```python
from build123d import *

# Parameters (mm, degrees)
EXTRUDE_THIN1_DEPTH = 698.5
FILLET2_R           = 1.27


with BuildPart() as part:
    # Sketch1 → Extrude-Thin1 (new body)
    with BuildSketch(Plane.XY):
        with BuildLine():
            Line((0, 0), (-11.1125, 0))
            Line((-11.1125, 0), (-11.1125, 12.7))
            Line((-11.1125, 12.7), (-8.73125, 12.7))
            Line((-8.73125, 12.7), (-8.73125, 19.05))
            ThreePointArc((-8.73125, 19.05), (-21.768435997, 25.910734502), (-26.9875, 39.6875))
            ThreePointArc((-26.9875, 39.6875), (-24.662660076, 45.300160076), (-19.05, 47.625))
            Line((-19.05, 47.625), (-19.05, 50.8))
            Line((-19.05, 50.8), (-26.9875, 50.8))
            Line((-26.9875, 50.8), (-26.9875, 69.85))
            Line((-26.9875, 69.85), (1.5875, 69.85))
            Line((1.5875, 69.85), (1.5875, 68.58))
            Line((1.5875, 68.58), (-25.7175, 68.58))
            Line((-25.7175, 68.58), (-25.7175, 52.07))
            Line((-25.7175, 52.07), (-17.78, 52.07))
            Line((-17.78, 52.07), (-17.78, 46.232930181))
            ThreePointArc((-17.78, 46.232930181), (-23.291923576, 44.831587929), (-25.7175, 39.6875))
            ThreePointArc((-25.7175, 39.6875), (-20.440161015, 26.338097436), (-7.46125, 20.205828325))
            Line((-7.46125, 20.205828325), (-7.46125, 11.43))
            Line((-7.46125, 11.43), (-9.8425, 11.43))
            Line((-9.8425, 11.43), (-9.8425, 1.27))
            Line((-9.8425, 1.27), (0, 1.27))
            Line((0, 1.27), (0, 0))
        make_face()
    extrude(amount=-EXTRUDE_THIN1_DEPTH)

    # Fillet2
    fillet2_edges = [part.edges().sort_by_distance(p)[0] for p in [
        (-17.78, 52.07, -349.25),
        (-17.78, 46.232930181, -349.25),
        (-7.46125, 20.205828325, -349.25),
        (-7.46125, 11.43, -349.25),
        (-11.1125, 0, -349.25),
        (-11.1125, 12.7, -349.25),
        (-26.9875, 50.8, -349.25),
        (-26.9875, 69.85, -349.25),
    ]]
    fillet(fillet2_edges, radius=FILLET2_R)


solid = part.part
```
Read the model definition and answer for the solid it produces. Units are mm, in the model's axes. A direction names the side the tool comes from. Give positions to 0.01 mm unless a question says otherwise; leave off trailing zeros. Loops run counter-clockwise (first coordinate to the right, second up) from the corner with the lowest first, then second, coordinate; pieces in that order, holes last.
Item 1: Find the intervals of material crossed by line 1 along Y through (x, z) = (-7, -520); line 2 along Y through (x, z) = (-21.25, -264); line 3 along Y through (x, z) = (-19, -640), in increasing order.
Item 2: Each of these flat-tipped pins is pushed along its axis until it touches: pin 1 Ø4 at (y, z) = (50.5, -372) entering from +X; pin 2 Ø1.6 at (y, z) = (49, -371.5) entering from -X; pin 3 Ø3 at (y, z) = (8, -288.5) entering from -X. Where does it stop, or does it pass through?
Item 3: The mould has two halves that part along Y. Classify faces 1 (the flat face through (-12, 69.85, -344)), 2 (the flat face through (-26.988, 60, -344)), 3 (the flat face through (-25.718, 60, -344)): released by +Y, released by -Y, zero draft, split by the parting line, or undercut.
Item 4: The part is cut by section B-B (y = 29). Write down the section's boundary in (x, z), and give its area (3 significant figures).
Item 5: For faces 4 (the flat face through (-18, 48, 0)), 5 (the cylindrical face through (-20.948, 26.901, -344.36)), determine the directions among +Z, -Z, +X, -X, +Y, -Y from which every point of the face is accessible in a straight line to the end or side of a thin tool.
Taken from the geometry:
1. line 1: y = 0 to 1.27, 68.58 to 69.85
1. line 2: y = 25.35 to 27.26, 45.98 to 47.31, 50.8 to 52.07, 68.58 to 69.85
1. line 3: y = 23.31 to 24.95, 46.36 to 52.07, 68.58 to 69.85
2. pin 1: stops at x = -17.78
2. pin 2: stops at x = -19.05
2. pin 3: stops at x = -11.11
3. face 1: released by +Y
3. face 2: zero draft
3. face 3: undercut
4. outline: (-24.03, -698.5) - (-22.53, -698.5) - (-22.53, 0) - (-24.03, 0) - close
4. area: 1,050 mm2
5. face 4: +Z, +X, -X, +Y, -Y
5. face 5: +Z, -Z, +X
